from build123d import *

# Parameters (mm, degrees)
SKETCH1_W           = 25.792857143
SKETCH1_H           = 6.35
SKETCH1_W_2         = 32.142857143
SKETCH1_W_3         = 6.35
SKETCH1_H_2         = 1.892857143
SKETCH1_H_3         = 8.242857143
BOSS_EXTRUDE1_DEPTH = 6.35
SKETCH2_W           = 225
SKETCH2_H           = 8.242857143
BOSS_EXTRUDE2_DEPTH = 6.35
SKETCH3_W           = 5.08
SKETCH3_H           = 6.35
BOSS_EXTRUDE3_DEPTH = 6.35
SKETCH4_W           = 20.32
SKETCH4_H           = 6.35
CUT_EXTRUDE1_DEPTH  = 6.35


with BuildPart() as part:
    # Sketch1 → Boss-Extrude1 (new body)
    with BuildSketch(Plane(origin=(0, 0, 0), x_dir=(1, 0, 0), z_dir=(0, 1, 0))):
        Polygon((6.35, 6.35), (32.142857143, 6.35), (64.285714286, 6.35), (96.428571429, 6.35), (128.571428571, 6.35), (160.714285714, 6.35), (192.857142857, 6.35), (218.65, 6.35), (218.65, 8.242857143), (218.65, 16.485714286), (218.65, 24.728571429), (218.65, 32.971428571), (218.65, 41.214285714), (218.65, 49.457142857), (218.65, 51.35), (192.857142857, 51.35), (160.714285714, 51.35), (128.571428571, 51.35), (96.428571429, 51.35), (64.285714286, 51.35), (32.142857143, 51.35), (6.35, 51.35), (6.35, 49.457142857), (6.35, 41.214285714), (6.35, 32.971428571), (6.35, 24.728571429), (6.35, 16.485714286), (6.35, 8.242857143), align=None)
        with Locations((19.246428572, 54.525)):
            Rectangle(SKETCH1_W, SKETCH1_H)
        with Locations((80.357142858, 54.525)):
            Rectangle(SKETCH1_W_2, SKETCH1_H)
        with Locations((144.642857143, 54.525)):
            Rectangle(SKETCH1_W_2, SKETCH1_H)
        with Locations((205.753571429, 54.525)):
            Rectangle(SKETCH1_W, SKETCH1_H)
        with Locations((221.825, 54.525)):
            Rectangle(SKETCH1_W_3, SKETCH1_H)
        with Locations((3.175, 54.525)):
            Rectangle(SKETCH1_W_3, SKETCH1_H)
        with Locations((3.175, 50.403571429)):
            Rectangle(SKETCH1_W_3, SKETCH1_H_2)
        with Locations((3.175, 7.296428571)):
            Rectangle(SKETCH1_W_3, SKETCH1_H_2)
        with Locations((3.175, 3.175)):
            Rectangle(SKETCH1_W_3, SKETCH1_H)
        with Locations((19.246428572, 3.175)):
            Rectangle(SKETCH1_W, SKETCH1_H)
        with Locations((80.357142858, 3.175)):
            Rectangle(SKETCH1_W_2, SKETCH1_H)
        with Locations((144.642857143, 3.175)):
            Rectangle(SKETCH1_W_2, SKETCH1_H)
        with Locations((205.753571429, 3.175)):
            Rectangle(SKETCH1_W, SKETCH1_H)
        with Locations((221.825, 3.175)):
            Rectangle(SKETCH1_W_3, SKETCH1_H)
        with Locations((221.825, 7.296428571)):
            Rectangle(SKETCH1_W_3, SKETCH1_H_2)
        with Locations((221.825, 50.403571429)):
            Rectangle(SKETCH1_W_3, SKETCH1_H_2)
        with Locations((221.825, 37.092857143)):
            Rectangle(SKETCH1_W_3, SKETCH1_H_3)
        with Locations((221.825, 20.607142858)):
            Rectangle(SKETCH1_W_3, SKETCH1_H_3)
        with Locations((3.175, 20.607142858)):
            Rectangle(SKETCH1_W_3, SKETCH1_H_3)
        with Locations((3.175, 37.092857143)):
            Rectangle(SKETCH1_W_3, SKETCH1_H_3)
    extrude(amount=BOSS_EXTRUDE1_DEPTH)

    # Sketch2 → Boss-Extrude2 (add)
    with BuildSketch(Plane(origin=(0, 6.35, 0), x_dir=(1, 0, 0), z_dir=(0, 1, 0))):
        with Locations((112.5, 53.578571428)):
            Rectangle(SKETCH2_W, SKETCH2_H)
    extrude(amount=-BOSS_EXTRUDE2_DEPTH)

    # Sketch3 → Boss-Extrude3 (add)
    with BuildSketch(Plane(origin=(0, 6.35, 0), x_dir=(1, 0, 0), z_dir=(0, 1, 0))):
        with Locations((23.6, 60.875)):
            Rectangle(SKETCH3_W, SKETCH3_H)
        with Locations((49, 60.875)):
            Rectangle(SKETCH3_W, SKETCH3_H)
        with Locations((74.4, 60.875)):
            Rectangle(SKETCH3_W, SKETCH3_H)
        with Locations((99.8, 60.875)):
            Rectangle(SKETCH3_W, SKETCH3_H)
        with Locations((125.2, 60.875)):
            Rectangle(SKETCH3_W, SKETCH3_H)
        with Locations((150.6, 60.875)):
            Rectangle(SKETCH3_W, SKETCH3_H)
        with Locations((176, 60.875)):
            Rectangle(SKETCH3_W, SKETCH3_H)
        with Locations((201.4, 60.875)):
            Rectangle(SKETCH3_W, SKETCH3_H)
    extrude(amount=-BOSS_EXTRUDE3_DEPTH)

    # Sketch4 → Cut-Extrude1 (cut)
    with BuildSketch(Plane(origin=(0, 6.35, 0), x_dir=(1, 0, 0), z_dir=(0, 1, 0))):
        with Locations((61.7, 54.525)):
            Rectangle(SKETCH4_W, SKETCH4_H)
        with Locations((36.3, 54.525)):
            Rectangle(SKETCH4_W, SKETCH4_H)
        with Locations((87.1, 54.525)):
            Rectangle(SKETCH4_W, SKETCH4_H)
        with Locations((112.5, 54.525)):
            Rectangle(SKETCH4_W, SKETCH4_H)
        with Locations((137.9, 54.525)):
            Rectangle(SKETCH4_W, SKETCH4_H)
        with Locations((163.3, 54.525)):
            Rectangle(SKETCH4_W, SKETCH4_H)
        with Locations((188.7, 54.525)):
            Rectangle(SKETCH4_W, SKETCH4_H)
    extrude(amount=-CUT_EXTRUDE1_DEPTH, mode=Mode.SUBTRACT)


solid = part.part
Geometry: final body of the model. Coordinates: model frame, mm. A direction names the side the tool comes from. Give positions to 0.01 mm unless a question says otherwise; leave off trailing zeros. Order: outer loops, then holes, each group sorted by start corner. A loop starts at its lowest first (then second) coordinate and runs counter-clockwise, first axis right, second up. Notation, with made-up numbers: (59.5, -25.75) -> (101.5, -25.75) arc R26 cw to (101.5, -0.75) -> close; hole circle Ø7 at (18.5, 21.5). An arc over 180 degrees is marked (long way). Write each question's results on one line, items separated by ' | '.
1) Cut plane B-B (x = 125). Output: boundary loops of the cut face in (y, z), and give its area (3 significant figures).
Geometry says:
outline: (0, -64.05) -> (6.35, -64.05) -> (6.35, -6.35) -> (0, -6.35) -> close | area: 366 mm²
2) First-contact query: pin 1 Ø1 at (x, y) = (161.5, 2.5) entering from +Z; pin 2 Ø1.9 at (y, z) = (2, -29) entering from -X; pin 3 Ø1.9 at (x, y) = (87.5, 4.5) entering from -Z. Flat tips, straight axial feed; report the tip coordinate or a pass-through.
Geometry says:
pin 1: stops at z = -6.35 | pin 2: stops at x = 6.35 | pin 3: stops at z = -51.35
3) Draft query along Z for faces 5 (the face through (225, 3, -4)), 6 (the face through (49, 3, -64.05)), 7 (the face through (3, 3, -8.243)). Return one class per face: released by +Z, released by -Z, zero draft, split by the parting line, or undercut.
Geometry says:
face 5: zero draft | face 6: released by -Z | face 7: undercut
4) Set-up query: faces 1 (the face through (3, 3, -24.729)), 2 (the face through (160.714, 3, -3)), 3 (the face through (203.94, 3, -61)), 4 (the face through (36, 3, -51.35)). Return all of +Z, -Z, +X, -X, +Y, -Y with unobstructed straight access to the full face (end or side cutting, diameter ignored); none if empty.
Geometry says:
face 1: -X, +Y, -Y | face 2: +Z, +Y, -Y | face 3: -Z, +X, +Y, -Y | face 4: -Z, +Y, -Y
5) Cut plane A-A (z = -55.5). Give the number of separate pieces and of enclosed holes in the cut face, and give its area (3 significant figures).
Geometry says:
separate pieces: 8 | enclosed holes: 0 | area: 526 mm²
6) Cut plane C-C (z = -12). Output: boundary loops of the cut face in (x, y).
Geometry says:
outline: (6.35, 0) -> (218.65, 0) -> (218.65, 6.35) -> (6.35, 6.35) -> close
7) Line query: line 1 along Z through (x, y) = (189.5, 5); line 2 along Z through (x, y) = (174, 5.5); line 3 along X through (y, z) = (5, -49). Output: solid intervals per line, ascending.
Geometry says:
line 1: z = -51.35 to -6.35 | line 2: z = -64.05 to -6.35 | line 3: x = 6.35 to 218.65
